Input: part model. Units: mm. Frame: model coordinates. Face numbers are marked on the shaded views. Round coordinates to 2 decimals unless told otherwise and drop trailing zeros. Loops run counter-clockwise (first coordinate to the right, second up) from the corner with the lowest first, then second, coordinate; pieces in that order, holes last.
1) Section A-A, the plane x = 40. Return loops of the section in (y, z).
2) First-contact query: pin 1 (8 mm diameter, centred on x = 457.5, y = 186.5, fed in from -Z); pin 2 (13 mm diameter, centred on y = 219.5, z = 43, fed in from -X); pin 3 (3 mm diameter, centred on y = 19, z = 54, fed in from -X); pin 4 (8 mm diameter, centred on x = 543, y = 187.5, fed in from +Z). Flat tips, straight axial feed; report the tip coordinate or a pass-through.
3) Section C-C, the plane z = 48. State how many separate pieces and enclosed holes the cut face has, and give its area (3 significant figures).
4) Section D-D, the plane x = 326. Return loops of the section in (y, z).
5) Section B-B, the plane y = 250. Return loops of the section in (x, z), and give its area (3 significant figures).
6) Draft query along Y for the marked faces 1, 2, 3 and 4. Return one class per face: pulls with the +Y half, pulls with the -Y half, needs draft (parallel to the pull), parting line crosses it, or undercut.
7) Ray query, line 1 along X through (y, z) = (15.75, 48); line 2 along Y through (x, z) = (312.5, 57); line 3 along Y through (x, z) = (764, 3). Return the intervals inside material, ascending.
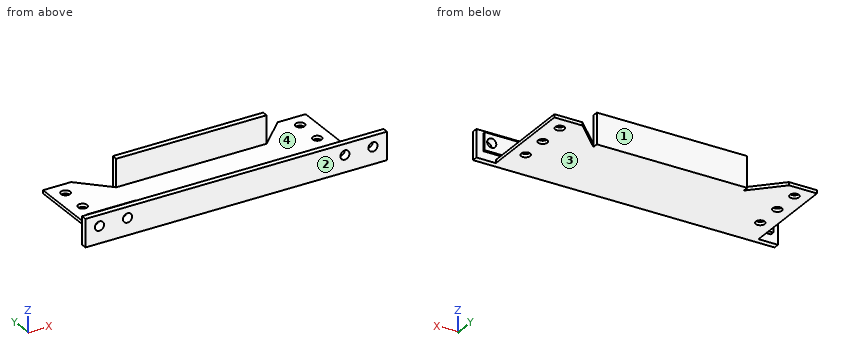
from build123d import *

# Parameters (mm, degrees)
SKETCH_1_R             = 13
EXTRUDE_2_DEPTH        = 9
SKETCH_3_W             = 860
SKETCH_3_H             = 16
EXTRUDE_3_DEPTH        = 70
SKETCH_4_W             = 140
SKETCH_4_H             = 50
EXTRUDE_5_DEPTH        = 11
SKETCH_5_R             = 13
CUT_EXTRUDE_2_DEPTH    = 903.779042734
PATTERN_LINEAR_1_COUNT = 2
PATTERN_LINEAR_1_PITCH = 80
SKETCH_6_W             = 140
SKETCH_6_H             = 50
EXTRUDE_6_DEPTH        = 6
SKETCH_7_R             = 13
CUT_EXTRUDE_3_DEPTH    = 905.248306606
PATTERN_LINEAR_2_COUNT = 2
PATTERN_LINEAR_2_PITCH = 80
SKETCH_10_W            = 429
SKETCH_10_H            = 16
EXTRUDE_8_DEPTH        = 79


with BuildPart() as part:
    # 草图1 → 凸台-拉伸2 (new body)
    with BuildSketch(Plane.XY):
        Polygon((0, 0), (860, 0), (860, 16), (804.5, 16), (804.5, 290), (724.5, 290), (644.5, 210), (644.5, 226), (215.5, 226), (215.5, 210), (135.5, 290), (55.5, 290), (55.5, 16), (0, 16), align=None)
        with Locations((95.5, 90)):
            Circle(SKETCH_1_R, mode=Mode.SUBTRACT)
        with Locations((95.5, 170)):
            Circle(SKETCH_1_R, mode=Mode.SUBTRACT)
        with Locations((95.5, 250)):
            Circle(SKETCH_1_R, mode=Mode.SUBTRACT)
        with Locations((764.5, 90)):
            Circle(SKETCH_1_R, mode=Mode.SUBTRACT)
        with Locations((764.5, 170)):
            Circle(SKETCH_1_R, mode=Mode.SUBTRACT)
        with Locations((764.5, 250)):
            Circle(SKETCH_1_R, mode=Mode.SUBTRACT)
    extrude(amount=EXTRUDE_2_DEPTH)

    # 草图3 → 凸台-拉伸3 (add)
    with BuildSketch(Plane.XY.offset(9)):
        with Locations((430, 8)):
            Rectangle(SKETCH_3_W, SKETCH_3_H)
    extrude(amount=EXTRUDE_3_DEPTH)

    # 草图4 → 凸台-拉伸5 (add)
    with BuildSketch(Plane(origin=(0, 16, 0), x_dir=(1, 0, 0), z_dir=(0, 1, 0))):
        with Locations((90, -48)):
            Rectangle(SKETCH_4_W, SKETCH_4_H)
    extrude(amount=EXTRUDE_5_DEPTH)

    # 草图5 → 切除-拉伸2 (cut, through all)
    with BuildSketch(Plane(origin=(0, 27, 0), x_dir=(1, 0, 0), z_dir=(0, 1, 0))):
        with Locations(Location((40, -48, 0), (0, 0, 270))):
            Circle(SKETCH_5_R)
    cut_extrude_2 = extrude(amount=-CUT_EXTRUDE_2_DEPTH, mode=Mode.SUBTRACT)

    # 阵列(线性)1: 切除-拉伸2 ×2
    with Locations(*[(i * PATTERN_LINEAR_1_PITCH, 0, 0) for i in range(1, PATTERN_LINEAR_1_COUNT)]):
        add(cut_extrude_2, mode=Mode.SUBTRACT)

    # 草图6 → 凸台-拉伸6 (add)
    with BuildSketch(Plane(origin=(0, 16, 0), x_dir=(1, 0, 0), z_dir=(0, 1, 0))):
        with Locations((770, -48)):
            Rectangle(SKETCH_6_W, SKETCH_6_H)
    extrude(amount=EXTRUDE_6_DEPTH)

    # 草图7 → 切除-拉伸3 (cut, through all)
    with BuildSketch(Plane(origin=(0, 22, 0), x_dir=(1, 0, 0), z_dir=(0, 1, 0))):
        with Locations(Location((820, -48, 0), (0, 0, 270))):
            Circle(SKETCH_7_R)
    cut_extrude_3 = extrude(amount=-CUT_EXTRUDE_3_DEPTH, mode=Mode.SUBTRACT)

    # 阵列(线性)2: 切除-拉伸3 ×2
    with Locations(*[(-i * PATTERN_LINEAR_2_PITCH, 0, 0) for i in range(1, PATTERN_LINEAR_2_COUNT)]):
        add(cut_extrude_3, mode=Mode.SUBTRACT)

    # 草图10 → 凸台-拉伸8 (add)
    with BuildSketch(Plane.XY.offset(9)):
        with Locations((430, 218)):
            Rectangle(SKETCH_10_W, SKETCH_10_H)
    extrude(amount=EXTRUDE_8_DEPTH)


solid = part.part
Final values:
1. outline: (0, 0) - (16, 0) - (16, 23) - (27, 23) - (27, 35) - (0, 35) - close; (0, 61) - (27, 61) - (27, 73) - (16, 73) - (16, 79) - (0, 79) - close
2. pin 1: stops at z = 0
2. pin 2: stops at x = 215.5
2. pin 3: stops at x = 20
2. pin 4: stops at z = 9
3. separate pieces: 6
3. enclosed holes: 0
3. area: 20,500 mm2
4. outline: (0, 0) - (226, 0) - (226, 88) - (210, 88) - (210, 9) - (16, 9) - (16, 79) - (0, 79) - close
5. outline: (55.5, 0) - (82.5, 0) - (82.5, 9) - (55.5, 9) - close; (108.5, 0) - (175.5, 0) - (175.5, 9) - (108.5, 9) - close; (684.5, 0) - (751.5, 0) - (751.5, 9) - (684.5, 9) - close; (777.5, 0) - (804.5, 0) - (804.5, 9) - (777.5, 9) - close
5. area: 1,690 mm2
6. face 1: pulls with the +Y half
6. face 2: pulls with the -Y half
6. face 3: needs draft
6. face 4: undercut
7. line 1: x = 0 to 27, 53 to 107, 133 to 727, 753 to 807, 833 to 860
7. line 2: y = 0 to 16, 210 to 226
7. line 3: y = 0 to 77.01, 102.99 to 157.01, 182.99 to 237.01, 262.99 to 290
